from build123d import *

# Parameters (mm, degrees)
SKETCH_1_W                   = 80
SKETCH_1_H                   = 100
EXTRUDE_1_DEPTH              = 3
SKETCH_2_W                   = 97
SKETCH_2_H                   = 57
SKETCH_2_W_2                 = 91
SKETCH_2_H_2                 = 51
EXTRUDE_2_DEPTH              = 45
SKETCH_3_W                   = 3
SKETCH_3_H                   = 34
EXTRUDE_3_DEPTH              = 51
SKETCH_4_W                   = 30
SKETCH_4_H                   = 6
CUT_EXTRUDE_2_DEPTH          = 50
SKETCH_5_W                   = 57
SKETCH_5_H                   = 57
SKETCH_5_W_2                 = 51
SKETCH_5_H_2                 = 51
EXTRUDE_4_DEPTH              = 30
HOLE_WIZARD_M3_1_D           = 2.5
HOLE_WIZARD_M3_1_CSINK_D     = 3.05
HOLE_WIZARD_M3_1_CSINK_ANGLE = 90
SKETCH_9_W                   = 3
SKETCH_9_H                   = 57
CUT_EXTRUDE_3_DEPTH          = 27


with BuildPart() as part:
    # 草图1 → 凸台-拉伸1 (new body)
    with BuildSketch(Plane(origin=(0, 0, 0), x_dir=(1, 0, 0), z_dir=(0, 1, 0))):
        with Locations((-20.765734509, -21.662442769)):
            Rectangle(SKETCH_1_W, SKETCH_1_H)
    extrude(amount=EXTRUDE_1_DEPTH)

    # 草图2 → 凸台-拉伸2 (add)
    with BuildSketch(Plane(origin=(0, 3, 0), x_dir=(1, 0, 0), z_dir=(0, 1, 0))):
        with Locations((-66.265734509, -21.662442769)):
            Rectangle(SKETCH_2_W, SKETCH_2_H)
        with Locations((-66.265734509, -21.662442769)):
            Rectangle(SKETCH_2_W_2, SKETCH_2_H_2, mode=Mode.SUBTRACT)
    extrude(amount=EXTRUDE_2_DEPTH)

    # 草图3 → 凸台-拉伸3 (add)
    with BuildSketch(Plane.XY.offset(-3.837557231)):
        with Locations((-73.265734509, 31)):
            Rectangle(SKETCH_3_W, SKETCH_3_H)
    extrude(amount=EXTRUDE_3_DEPTH)

    # 草图4 → 切除-拉伸2 (cut)
    with BuildSketch(Plane(origin=(0, 0, -6.837557231), x_dir=(-1, 0, 0), z_dir=(0, 0, -1))):
        with Locations((32.765734509, 6)):
            Rectangle(SKETCH_4_W, SKETCH_4_H)
    extrude(amount=-CUT_EXTRUDE_2_DEPTH, mode=Mode.SUBTRACT)

    # 草图5 → 凸台-拉伸4 (add)
    with BuildSketch(Plane.XZ.offset(-3)):
        with Locations((-86.265734509, 21.662442769)):
            Rectangle(SKETCH_5_W, SKETCH_5_H)
        with Locations((-86.265734509, 21.662442769)):
            Rectangle(SKETCH_5_W_2, SKETCH_5_H_2, mode=Mode.SUBTRACT)
    extrude(amount=EXTRUDE_4_DEPTH)

    # M3 螺纹孔1 (through all)
    with Locations(Plane(origin=(0, 3, 0), x_dir=(1, 0, 0), z_dir=(0, 1, 0))):
        with Locations((-46.765734509, 18.337557231), (13.234265491, 18.337557231), (13.234265491, -61.662442769), (-46.765734509, -61.662442769)):
            CounterSinkHole(HOLE_WIZARD_M3_1_D / 2, HOLE_WIZARD_M3_1_CSINK_D / 2, counter_sink_angle=HOLE_WIZARD_M3_1_CSINK_ANGLE)

    # 草图9 → 切除-拉伸3 (cut)
    with BuildSketch(Plane(origin=(0, -27, 0), x_dir=(-1, 0, 0), z_dir=(0, -1, 0))):
        with Locations((59.265734509, -21.662442769)):
            Rectangle(SKETCH_9_W, SKETCH_9_H)
    extrude(amount=-CUT_EXTRUDE_3_DEPTH, mode=Mode.SUBTRACT)


solid = part.part
Can you work these out from the model? Positions are in its coordinate system, mm. A direction names the side the tool comes from. Give positions to 0.01 mm unless a question says otherwise; leave off trailing zeros. Write each loop counter-clockwise with the first axis right and the second up, starting at its lowest first coordinate (ties: lowest second). Pieces come first, ordered by that corner, then holes. Notation, with made-up numbers: M -15,54 L 32,54 A15 cw 32,63 Z; hole C 69,-2.5 d8. An arc over 180 degrees is marked long. Answer in a Markdown table with one row per item. Add a question column.
Item 1: On a 3-axis mill with a long thin cutter (end or side, diameter ignored), from which of +Z, -Z, +X, -X, +Y, -Y can I reach the whole of each face in a straight line? I mean faces 4 (the flat face through (-20, 0, 21)), 5 (the flat face through (-60.766, 1, 61)), 6 (the flat face through (-20.766, 25, 22)), 7 (the flat face through (-60.766, 1, -17)), 8 (the flat face through (-73, 14, 21)). Say none if no direction works.
Item 2: Imagine slicing it at A-A, the plane x = -81.5. Write out the boundary of the cut face in (y, z).
Item 3: Imagine slicing it at D-D, the plane x = -38.5. Write out the boundary of the cut face in (y, z), plus the area to 3 significant figures.
Item 4: We'd pull the mould along Z, two halves only. Please class faces 1 (the flat face through (-21, 1, -28.338)), 2 (the flat face through (-60.766, 2, 21)), 3 (the flat face through (-74, 48, 22)): released by +Z, released by -Z, zero draft, split by the parting line, or undercut.
Item 5: Imagine slicing it at C-C, the plane y = 40. Write out the boundary of the cut face in (x, z).
Item 6: Imagine slicing it at B-B, the plane z = 38.5. Write out the boundary of the cut face in (x, y).
Item 7: Please list where these lines run through material, in increasing order: L1, parallel to X at y = 16, z = 24; L2, parallel to Z at x = -59, y = 7.5; L3, parallel to Y at x = -17.5, z = -3.5.
Item 8: For pin 1 Ø22.5 at (x, y) = (-83.5, 18) entering from -Z; pin 2 Ø3 at (x, z) = (-46.77, -18.34) entering from -Y; pin 3 Ø5 at (y, z) = (0, -7.5) entering from -X; pin 4 Ø1.5 at (y, z) = (-17, 49.5) entering from +X, each with a flat end and sliding along its axis, tell me the tip position at first contact or that it passes through.
Evaluation:
| question | item | result |
|---|---|---|
| 1 | face 4 | +Z, -Z, +X, -Y |
| 1 | face 5 | +Z, -X, +Y, -Y |
| 1 | face 6 | +Y |
| 1 | face 7 | -Z, -X, +Y, -Y |
| 1 | face 8 | -Y |
| 2 | outline | M -27,-6.84 L 48,-6.84 L 48,-3.84 L -27,-3.84 Z; M -27,47.16 L 48,47.16 L 48,50.16 L -27,50.16 Z |
| 3 | outline | M 0,-28.34 L 3,-28.34 L 3,47.16 L 48,47.16 L 48,50.16 L 3,50.16 L 3,71.66 L 0,71.66 Z; M 9,-6.84 L 48,-6.84 L 48,-3.84 L 9,-3.84 Z |
| 3 | area | 552 mm² |
| 4 | face 1 | released by -Z |
| 4 | face 2 | undercut |
| 4 | face 3 | zero draft |
| 5 | outline | M -114.77,-6.84 L -17.77,-6.84 L -17.77,50.16 L -114.77,50.16 Z; hole M -111.77,-3.84 L -74.77,-3.84 L -74.77,47.16 L -111.77,47.16 Z; hole M -71.77,-3.84 L -20.77,-3.84 L -20.77,47.16 L -71.77,47.16 Z |
| 6 | outline | M -114.77,-27 L -111.77,-27 L -111.77,48 L -114.77,48 Z; M -74.77,14 L -71.77,14 L -71.77,48 L -74.77,48 Z; M -60.77,0 L 19.23,0 L 19.23,3 L -60.77,3 Z; M -20.77,9 L -17.77,9 L -17.77,48 L -20.77,48 Z |
| 7 | L1 | x = -114.77 to -111.77, -74.77 to -71.77, -20.77 to -17.77 |
| 7 | L2 | z = -6.84 to -3.84, 47.16 to 50.16 |
| 7 | L3 | y = 0 to 3 |
| 8 | pin 1 | stops at z = -6.84 |
| 8 | pin 2 | stops at y = 0 |
| 8 | pin 3 | stops at x = -114.77 |
| 8 | pin 4 | stops at x = -60.77 |
